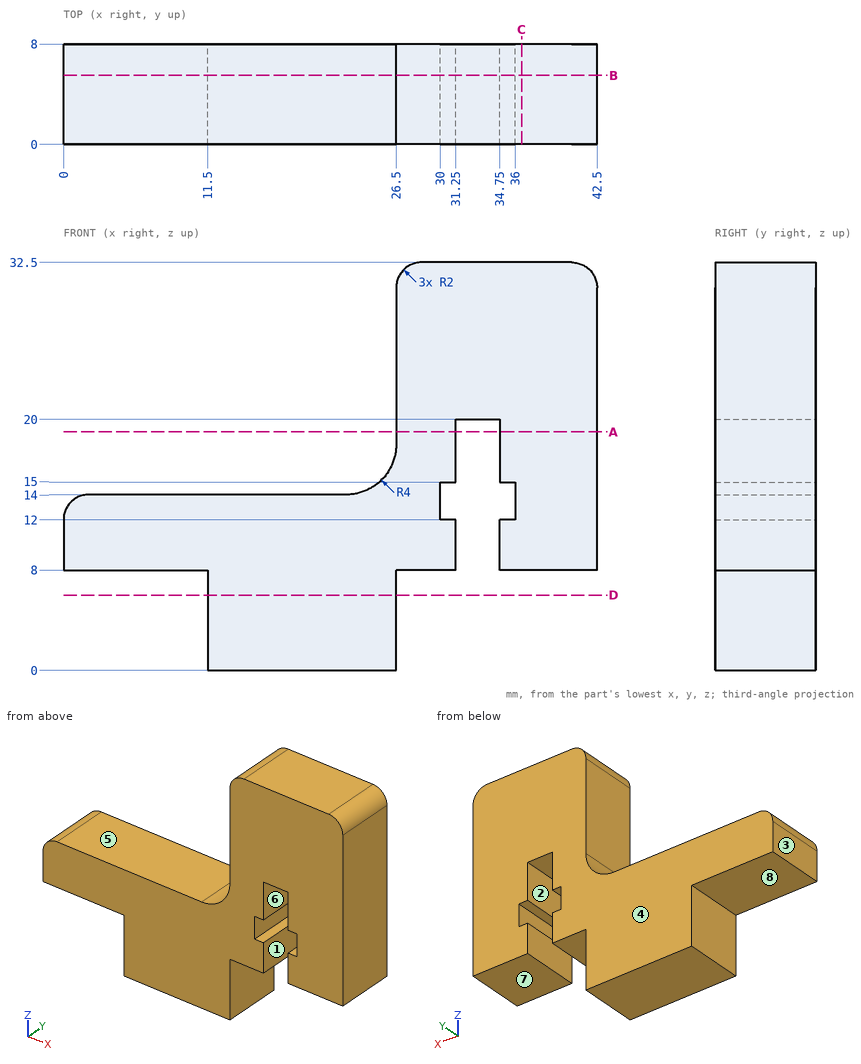
The drawing under review shows one solid part. Ordinate dimensions are in mm from its lowest x, y, z. A direction names the side the tool comes from. Round coordinates to 2 decimals unless told otherwise and drop trailing zeros. Loops run counter-clockwise (first coordinate to the right, second up) from the corner with the lowest first, then second, coordinate; pieces in that order, holes last. Notation, with made-up numbers: (-1, -24.5) -> (18, -24.5) arc R21 cw to (18, -3.5) -> close; hole circle Ø9 at (-26.75, 0.5). An arc over 180 degrees is marked (long way). One line per question, with ' | ' between items. Start each with the question number.
Item 1: Add section D-D, the plane z = 6. Write out the cut boundary in (x, y).
Item 2: Add section B-B, the plane y = 5.5. Write out the cut boundary in (x, z), then the cut area to 3 significant figures.
Item 3: Machinability: for the marked faces 5, 6, 7 and 8, which of the approach directions +Z, -Z, +X, -X, +Y, -Y give a long, thin tool a straight path to every point of the face, cutting with its end or side? Answer none if there is none.
Item 4: For pin 1 (4 mm diameter, centred on y = 3, z = 24.5, fed in from -X); pin 2 (4 mm diameter, centred on y = 7, z = 8.5, fed in from -X); pin 3 (1 mm diameter, centred on x = 35.5, y = 4, fed in from -Z); pin 4 (1 mm diameter, centred on x = 25.5, y = 6.5, fed in from +Z), all flat-tipped, find the tip position at first contact; note any pin that passes through.
Item 5: Draft analysis for pull direction X (two halves, no side actions). For the marked faces 1, 2, 3 and 4, state which applies: +X half, -X half, draft (parallel to the pull), parting line (faces both ways), or undercut.
Item 6: Add section C-C, the plane x = 36.5. Write out the cut boundary in (y, z).
Item 7: Wall thickness on line 1 along X through (y, z) = (3.25, 10.5); line 2 along X through (y, z) = (5.5, 6); line 3 along Z through (x, y) = (13, 5.25): over which ranges is each line inside the solid? List them lowest first. Write a range as [from, to].
Item 8: Add section A-A, the plane z = 19. Write out the cut boundary in (x, y), then the cut area to 3 significant figures.
Return value:
1) outline: (11.5, 0) -> (26.5, 0) -> (26.5, 8) -> (11.5, 8) -> close
2) outline: (0, 8) -> (11.5, 8) -> (11.5, 0) -> (26.5, 0) -> (26.5, 8) -> (31.25, 8) -> (31.25, 12) -> (30, 12) -> (30, 15) -> (31.25, 15) -> (31.25, 20) -> (34.75, 20) -> (34.75, 15) -> (36, 15) -> (36, 12) -> (34.75, 12) -> (34.75, 8) -> (42.5, 8) -> (42.5, 30.5) arc R2 ccw to (40.5, 32.5) -> (28.5, 32.5) arc R2 ccw to (26.5, 30.5) -> (26.5, 18) arc R4 cw to (22.5, 14) -> (2, 14) arc R2 ccw to (0, 12) -> close | area: 622 mm2
3) face 5: +Z, -X, +Y, -Y | face 6: -Z, +Y, -Y | face 7: -Z, +X, +Y, -Y | face 8: -Z, -X, +Y, -Y
4) pin 1: stops at x = 26.5 | pin 2: stops at x = 0 | pin 3: stops at z = 8 | pin 4: stops at z = 16.06
5) face 1: undercut | face 2: undercut | face 3: -X half | face 4: draft
6) outline: (0, 8) -> (8, 8) -> (8, 32.5) -> (0, 32.5) -> close
7) line 1: x = [0, 31.25], [34.75, 42.5] | line 2: x = [11.5, 26.5] | line 3: z = [0, 14]
8) outline: (26.5, 0) -> (31.25, 0) -> (31.25, 8) -> (26.5, 8) -> close; (34.75, 0) -> (42.5, 0) -> (42.5, 8) -> (34.75, 8) -> close | area: 100 mm2
